```python
from build123d import *

# Parameters (mm, degrees)
SKETCH_1_W          = 13
SKETCH_1_H          = 26
EXTRUDE_1_DEPTH     = 2.5
SKETCH_2_R          = 1.6
CUT_EXTRUDE_1_DEPTH = 13
SKETCH_3_W          = 13
SKETCH_3_H          = 5
EXTRUDE_2_DEPTH     = 24
SKETCH_4_W          = 13
SKETCH_4_H          = 12
EXTRUDE_3_DEPTH     = 43
SKETCH_5_W          = 3.5
SKETCH_5_H          = 25
EXTRUDE_4_DEPTH     = 48
SKETCH_6_R          = 0.91
SKETCH_6_R_2        = 0.9
CUT_EXTRUDE_2_DEPTH = 16
SKETCH_7_W          = 18
SKETCH_7_H          = 8
CUT_EXTRUDE_3_DEPTH = 16


with BuildPart() as part:
    # 草图1 → 凸台-拉伸1 (new, symmetric)
    with BuildSketch(Plane(origin=(0, 0, 0), x_dir=(1, 0, 0), z_dir=(0, 1, 0))):
        Rectangle(SKETCH_1_W, SKETCH_1_H)
    extrude(amount=EXTRUDE_1_DEPTH, both=True)

    # 草图2 → 切除-拉伸1 (cut)
    with BuildSketch(Plane(origin=(0, 2.5, 0), x_dir=(1, 0, 0), z_dir=(0, 1, 0))):
        with Locations(Location((0, 9.4, 0), (0, 0, 270))):
            Circle(SKETCH_2_R)
        with Locations(Location((0, -9.4, 0), (0, 0, 270))):
            Circle(SKETCH_2_R)
    extrude(amount=-CUT_EXTRUDE_1_DEPTH, mode=Mode.SUBTRACT)

    # 草图3 → 凸台-拉伸2 (add)
    with BuildSketch(Plane.XY.offset(13)):
        Rectangle(SKETCH_3_W, SKETCH_3_H)
    extrude(amount=EXTRUDE_2_DEPTH)

    # 草图4 → 凸台-拉伸3 (add)
    with BuildSketch(Plane.XZ.offset(2.5)):
        with Locations((0, 31)):
            Rectangle(SKETCH_4_W, SKETCH_4_H)
    extrude(amount=EXTRUDE_3_DEPTH)

    # 草图5 → 凸台-拉伸4 (add)
    with BuildSketch(Plane.ZY.offset(6.5)):
        with Locations((35.25, -33)):
            Rectangle(SKETCH_5_W, SKETCH_5_H)
    extrude(amount=EXTRUDE_4_DEPTH)

    # 草图6 → 切除-拉伸2 (cut)
    with BuildSketch(Plane.XY.offset(37)):
        with Locations((-51.5, -23.5)):
            Circle(SKETCH_6_R)
        with Locations((-8.68, -23.5)):
            Circle(SKETCH_6_R_2)
        with Locations((-51.5, -41.24)):
            Circle(SKETCH_6_R)
        with Locations((-8.68, -41.24)):
            Circle(SKETCH_6_R)
    extrude(amount=-CUT_EXTRUDE_2_DEPTH, mode=Mode.SUBTRACT)

    # 草图7 → 切除-拉伸3 (cut)
    with BuildSketch(Plane.XY.offset(37)):
        with Locations((-30.09, -24.5)):
            Rectangle(SKETCH_7_W, SKETCH_7_H)
        with Locations((-30.09, -41.5)):
            Rectangle(SKETCH_7_W, SKETCH_7_H)
    extrude(amount=-CUT_EXTRUDE_3_DEPTH, mode=Mode.SUBTRACT)


solid = part.part
```
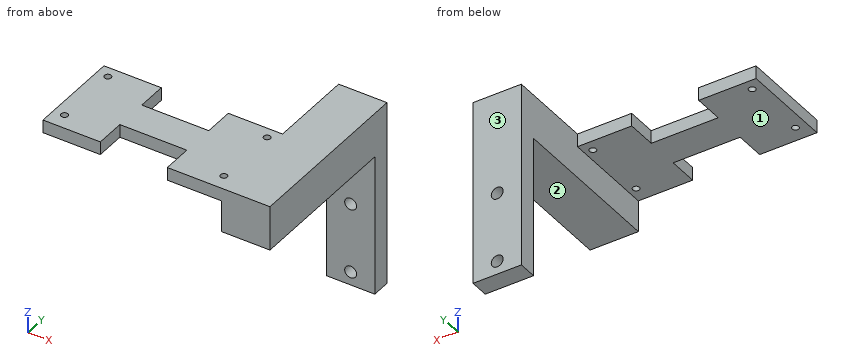
Could you check a few things on this model? Use its own coordinates, in mm. Face numbers are marked on the shaded views. A direction names the side the tool comes from. Coordinates: 2 decimals unless noted, no trailing zeros. Order: outer loops, then holes, each group sorted by start corner. A loop starts at its lowest first (then second) coordinate and runs counter-clockwise, first axis right, second up. Notation, with made-up numbers: M 60.25,39.5 L 77.25,39.5 A25 ccw 77.25,58.5 Z; hole C 55.25,16.25 d2. An arc over 180 degrees is marked long. Use a Markdown table: item, result. Add a question column.
Q1. I want a section at A-A on x = -8.68. List the corners of the cut face in (y, z) for me.
Q2. Which directions (+Z, -Z, +X, -X, +Y, -Y) give clear straight access to the entire face, cutting with the end or side of a thin tool? Please do the marked faces 1, 2 and 3.
Q3. I want a section at D-D on x = 0. List the corners of the cut face in (y, z) for me, then the cut area to 3 significant figures.
Q4. If I drill on L1, parallel to Y at x = -51.5, z = 34.6; L2, parallel to X at y = -41, z = 35; L3, parallel to X at y = -4.5, z = 33, over which ranges is the centre line in solid material (lowest first)?
Q5. I want a section at B-B on z = -9.4. List the corners of the cut face in (x, y) for me.
Q6. I want a section at C-C on y = -23.5. List the corners of the cut face in (x, z) for me, then the cut area to 3 significant figures.
Q7. I'm going to push flat-ended pins straight in: pin 1 (1 mm diameter, centred on x = -27, z = 35.5, fed in from -Y); pin 2 (6 mm diameter, centred on x = -4, y = -5, fed in from -Z); pin 3 (8 mm diameter, centred on y = -9.5, z = -8, fed in from +X); pin 4 (14.5 mm diameter, centred on x = -2, z = 9, fed in from -Y). Where does each tip first touch, or does it pass through?
Checked values:
| question | item | result |
|---|---|---|
| 1 | outline | M -45.5,33.5 L -42.15,33.5 L -42.15,37 L -45.5,37 Z; M -40.33,33.5 L -24.4,33.5 L -24.4,37 L -40.33,37 Z; M -22.6,33.5 L -20.5,33.5 L -20.5,37 L -22.6,37 Z |
| 2 | face 1 | -Z, -X, +Y, -Y |
| 2 | face 2 | -Z, +X, -X, -Y |
| 2 | face 3 | +Z, -Z, +X, -X, +Y |
| 3 | outline | M -45.5,25 L -2.5,25 L -2.5,11 L 2.5,11 L 2.5,37 L -45.5,37 Z; M -2.5,-13 L 2.5,-13 L 2.5,-11 L -2.5,-11 Z; M -2.5,-7.8 L 2.5,-7.8 L 2.5,7.8 L -2.5,7.8 Z |
| 3 | area | 734 mm² |
| 4 | L1 | -45.5 to -42.15, -40.33 to -24.41, -22.59 to -20.5 |
| 4 | L2 | -54.5 to -52.38, -50.62 to -39.09, -21.09 to -9.56, -7.8 to 6.5 |
| 4 | L3 | -6.5 to 6.5 |
| 5 | outline | M -6.5,-2.5 L -1.6,-2.5 L -1.6,2.5 L -6.5,2.5 Z; M 1.6,-2.5 L 6.5,-2.5 L 6.5,2.5 L 1.6,2.5 Z |
| 6 | outline | M -54.5,33.5 L -52.41,33.5 L -52.41,37 L -54.5,37 Z; M -50.59,33.5 L -39.09,33.5 L -39.09,37 L -50.59,37 Z; M -21.09,33.5 L -9.58,33.5 L -9.58,37 L -21.09,37 Z; M -7.78,33.5 L -6.5,33.5 L -6.5,25 L 6.5,25 L 6.5,37 L -7.78,37 Z |
| 6 | area | 248 mm² |
| 7 | pin 1 | y = -37.5 |
| 7 | pin 2 | z = -13 |
| 7 | pin 3 | through |
| 7 | pin 4 | y = -2.5 |
